```python
from build123d import *

# Parameters (mm, degrees)
BOSS_EXTRUDE1_DEPTH                               = 5.08
BOSS_EXTRUDE1_DEPTH_BACK                          = 5.08
SKETCH2_R                                         = 1.5875
CUT_EXTRUDE1_DEPTH                                = 3.175
CUT_EXTRUDE1_DEPTH_BACK                           = 11.557
CHAMFER1_SIZE                                     = 2.54
CHAMFER2_SIZE                                     = 2.54
CSK_FOR_6_FLAT_HEAD_MACHINE_SCREW_100_D           = 3.7973
CSK_FOR_6_FLAT_HEAD_MACHINE_SCREW_100_CSINK_D     = 7.0866
CSK_FOR_6_FLAT_HEAD_MACHINE_SCREW_100_CSINK_ANGLE = 100
SKETCH6_W                                         = 67.564
SKETCH6_H                                         = 10.16
SKETCH6_R                                         = 1.89865
BOSS_EXTRUDE2_DEPTH                               = 2.54
SKETCH7_R                                         = 1.5875
CUT_EXTRUDE2_DEPTH                                = 6.08
CUT_EXTRUDE2_DEPTH_BACK                           = 6.08


with BuildPart() as part:
    # Sketch1 → Boss-Extrude1 (new body, two sides)
    with BuildSketch(Plane.XY) as boss_extrude1_sk:
        Polygon((30.2895, 0.070457444), (-0.3175, 0.070457444), (-30.9245, 0.070457444), (-30.9245, 15.310457444), (-29.0195, 16.51), (-30.711281219, 19.196726876), (-34.0995, 17.06322944), (-34.0995, -3.104542556), (33.4645, -3.104542556), (33.4645, 17.06322944), (30.076281219, 19.196726876), (28.3845, 16.51), (30.2895, 15.310457444), align=None)
    extrude(amount=BOSS_EXTRUDE1_DEPTH)
    extrude(boss_extrude1_sk.sketch, amount=-BOSS_EXTRUDE1_DEPTH_BACK)

    # Sketch2 → Cut-Extrude1 (cut, two sides)
    with BuildSketch(Plane(origin=(0, 0, 0), x_dir=(1, 0, 0), z_dir=(0, 1, 0))) as cut_extrude1_sk:
        with Locations((-12.954, 0)):
            Circle(SKETCH2_R)
        with Locations((12.954, 0)):
            Circle(SKETCH2_R)
    extrude(amount=CUT_EXTRUDE1_DEPTH, mode=Mode.SUBTRACT)
    extrude(cut_extrude1_sk.sketch, amount=-CUT_EXTRUDE1_DEPTH_BACK, mode=Mode.SUBTRACT)

    # Chamfer1
    chamfer1_edges = [part.edges().sort_by_distance(p)[0] for p in [
        (30.2895, 0.070457444, 0),
    ]]
    chamfer(chamfer1_edges, length=CHAMFER1_SIZE)

    # Chamfer2
    chamfer2_edges = [part.edges().sort_by_distance(p)[0] for p in [
        (-30.9245, 0.070457444, 0),
    ]]
    chamfer(chamfer2_edges, length=CHAMFER2_SIZE)

    # CSK for #6 Flat Head Machine Screw (100)2 (through all)
    with Locations(Plane(origin=(-12.954, 0.070457444, 0), x_dir=(1, 0, 0), z_dir=(0, 1, 0))):
        with Locations((0, 0), (25.908, 0)):
            CounterSinkHole(CSK_FOR_6_FLAT_HEAD_MACHINE_SCREW_100_D / 2, CSK_FOR_6_FLAT_HEAD_MACHINE_SCREW_100_CSINK_D / 2, counter_sink_angle=CSK_FOR_6_FLAT_HEAD_MACHINE_SCREW_100_CSINK_ANGLE)

    # Sketch6 → Boss-Extrude2 (add)
    with BuildSketch(Plane(origin=(0, -3.104542556, 0), x_dir=(-1, 0, 0), z_dir=(0, -1, 0))):
        with Locations((0.3175, 0)):
            Rectangle(SKETCH6_W, SKETCH6_H)
        with Locations((12.954, 0)):
            Circle(SKETCH6_R, mode=Mode.SUBTRACT)
        with Locations((-12.954, 0)):
            Circle(SKETCH6_R, mode=Mode.SUBTRACT)
    extrude(amount=BOSS_EXTRUDE2_DEPTH)

    # Sketch7 → Cut-Extrude2 (cut, two sides)
    with BuildSketch(Plane.XY) as cut_extrude2_sk:
        with Locations((19.200527544, -2.787042556)):
            Circle(SKETCH7_R)
    extrude(amount=CUT_EXTRUDE2_DEPTH, mode=Mode.SUBTRACT)
    extrude(cut_extrude2_sk.sketch, amount=-CUT_EXTRUDE2_DEPTH_BACK, mode=Mode.SUBTRACT)


solid = part.part
```
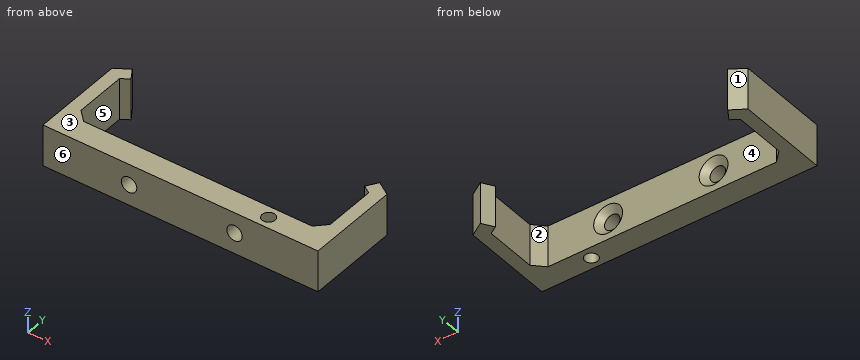
Geometry check sheet. Reference: the model listing, model coordinates, mm. Face numbers are marked on the shaded views. A direction names the side the tool comes from. Give positions to 0.01 mm unless a question says otherwise; leave off trailing zeros. Order: outer loops, then holes, each group sorted by start corner. A loop starts at its lowest first (then second) coordinate and runs counter-clockwise, first axis right, second up. Notation, with made-up numbers: (76, -19.75) - (104, -19.75) arc R16 ccw to (104, -14.75) - close; hole circle Ø9 at (71, -17.75). An arc over 180 degrees is marked (long way). Answer in a Markdown table with one row per item. Add a question column.
Q1. Material ranges on probe 1 along X at (y, z) = (-4.5, 0); probe 2 along X at (y, z) = (4.5, -0.25); probe 3 along X at (y, z) = (-4.1, 0), recorded low to high. Write a range as from..to.
Q2. Mould release check, pull along Y, two halves, no side actions. Record for the marked faces 1, 2 and 3: pulls with the +Y half, pulls with the -Y half, needs draft (parallel to the pull), parting line crosses it, or undercut.
Q3. Tool access check on the marked faces 4, 5 and 6. Record the directions out of +Z, -Z, +X, -X, +Y, -Y that give a thin tool (end or side, any length) a straight path to the whole face; none if there is none.
Q4. Cross-section at D-D, the plane x = 2.5. Enter the section's corners in (y, z), then the cut area to 3 significant figures.
Q5. Cross-section at B-B, the plane y = 11.75. Enter the section's corners in (x, z), then the cut area to 3 significant figures.
Q6. Gauge pin test, flat ends, axial feed: pin 1 (3 mm diameter, centred on x = 19.2, y = -2.79, fed in from -Z); pin 2 (4 mm diameter, centred on x = -0.5, z = -3, fed in from +Y). Record the tip position at first contact, or that the pin passes through.
Q7. Cross-section at A-A, the plane z = 0. Enter the section's corners in (x, y) (1 decimal).
Q8. Cross-section at C-C, the plane y = -2. Enter the section's corners in (x, z), then the cut area to 3 significant figures.
Check values:
| question | item | result |
|---|---|---|
| 1 | probe 1 | x = -34.1..-14.85, -11.06..11.06, 14.85..33.46 |
| 1 | probe 2 | x = -34.1..-30.92, 30.29..33.46 |
| 1 | probe 3 | x = -34.1..-14.85, -11.06..11.06, 14.85..18.31, 20.09..33.46 |
| 2 | face 1 | pulls with the +Y half |
| 2 | face 2 | undercut |
| 2 | face 3 | needs draft |
| 3 | face 4 | +Z, -Z, +Y |
| 3 | face 5 | +Z, -Z |
| 3 | face 6 | +Z, -Z, +X, -X, -Y |
| 4 | outline | (-5.64, -5.08) - (0.07, -5.08) - (0.07, 5.08) - (-5.64, 5.08) - close |
| 4 | area | 58.1 mm^2 |
| 5 | outline | (-34.1, -5.08) - (-30.92, -5.08) - (-30.92, 5.08) - (-34.1, 5.08) - close; (30.29, -5.08) - (33.46, -5.08) - (33.46, 5.08) - (30.29, 5.08) - close |
| 5 | area | 64.5 mm^2 |
| 6 | pin 1 | passes through |
| 6 | pin 2 | stops at y = 0.07 |
| 7 | outline | (-34.1, -5.6) - (-14.9, -5.6) - (-14.9, -1.3) - (-16.5, 0.1) - (-28.4, 0.1) - (-30.9, 2.6) - (-30.9, 15.3) - (-29, 16.5) - (-30.7, 19.2) - (-34.1, 17.1) - close; (-11.1, -5.6) - (11.1, -5.6) - (11.1, -1.3) - (9.4, 0.1) - (-9.4, 0.1) - (-11.1, -1.3) - close; (14.9, -5.6) - (33.5, -5.6) - (33.5, 17.1) - (30.1, 19.2) - (28.4, 16.5) - (30.3, 15.3) - (30.3, 2.6) - (27.7, 0.1) - (16.5, 0.1) - (14.9, -1.3) - close; hole circle Ø3.2 at (19.2, -2.8) |
| 8 | outline | (-34.1, -5.08) - (17.82, -5.08) - (17.82, 5.08) - (-34.1, 5.08) - close; (20.58, -5.08) - (33.46, -5.08) - (33.46, 5.08) - (20.58, 5.08) - close; hole circle Ø3.8 at (-12.95, 0); hole circle Ø3.8 at (12.95, 0) |
| 8 | area | 636 mm^2 |
